Part model, mm, in its own coordinate system. A direction names the side the tool comes from. Round coordinates to 2 decimals unless told otherwise and drop trailing zeros. Write each loop counter-clockwise with the first axis right and the second up, starting at its lowest first coordinate (ties: lowest second). Pieces come first, ordered by that corner, then holes. Notation, with made-up numbers: M -2.5,86.25 L 29.5,86.25 A26 ccw 29.5,102.25 Z; hole C 34.25,8.25 d4. An arc over 180 degrees is marked long. Answer as a JSON object with one key per item and string values. Group by question number.
1. Band-saw the part on A-A, the plane y = 40.5. Write the cut outline in (x, z), plus the area to 3 significant figures.
2. Drill centre lines: line 1 (Y direction, x = -40, z = 34); line 2 (Y direction, x = 34.5, z = 29.5). Where is each one in solid material? Low to high. Write a range as from..to.
3. Two-plate mould, pull along X, no slides. Class faces 1 (the face through (40, -40, 32)), 2 (the face through (44, -1, 21)), 3 (the face through (-1, -44, 21)): +X half, -X half, draft (parallel to the pull), parting line (faces both ways), or undercut.
4. Band-saw the part on D-D, the plane z = 38.5. Write the cut outline in (x, y).
5. Band-saw the part on B-B, the plane x = 22.5. Write the cut outline in (y, z), plus the area to 3 significant figures.
6. Band-saw the part on C-C, the plane z = 9.5. Write the cut outline in (x, y), plus the area to 3 significant figures.
7. Which spindle directions (+Z, -Z, +X, -X, +Y, -Y) get a long thin tool onto all of the face, cutting with end or side? Do faces 4 (the face through (37.19, -40, 22)), 5 (the face through (-1, 44, 21)). Say none if no direction does.
8. Drop a flat-ended pin along its axis: pin 1 (0.8 mm diameter, centred on x = -40.5, y = -40.5, fed in from +Z). Give the stop position or say it passes through.
from build123d import *

# Parameters (mm, degrees)
SKETCH_W        = 88
SKETCH_H        = 88
PAD_DEPTH       = 42
SKETCH001_W     = 84
SKETCH001_H     = 84
POCKET_DEPTH    = 39
SKETCH002_W     = 5
SKETCH002_H     = 5
PAD001_DEPTH    = 39
SKETCH003_R     = 1.25
POCKET001_DEPTH = 10


with BuildPart() as part:
    # Sketch → Pad (new body)
    with BuildSketch(Plane.XY):
        Rectangle(SKETCH_W, SKETCH_H)
    extrude(amount=PAD_DEPTH)

    # Sketch001 (on Face6 of Pad) → Pocket (cut)
    with BuildSketch(Plane.XY.offset(42)):
        Rectangle(SKETCH001_W, SKETCH001_H)
    extrude(amount=-POCKET_DEPTH, mode=Mode.SUBTRACT)

    # Sketch002 (on Face11 of Pocket) → Pad001 (join)
    with BuildSketch(Plane.XY.offset(3)):
        with Locations((-39.556091, 39.69)):
            Rectangle(SKETCH002_W, SKETCH002_H)
        with Locations((-39.69, -39.556091)):
            Rectangle(SKETCH002_W, SKETCH002_H)
    pad001 = extrude(amount=PAD001_DEPTH)

    # Mirrored: Pad001 across Sketch002 V_Axis
    add(pad001.mirror(Plane(origin=(0, 0, 3), x_dir=(0, 0, 1), z_dir=(1, 0, 0))))

    # Sketch003 (on Face6 of Mirrored) → Pocket001 (cut)
    with BuildSketch(Plane.XY.offset(42)):
        with Locations((-40, 40.5)):
            Circle(SKETCH003_R)
        with Locations((-40, -40.5)):
            Circle(SKETCH003_R)
    pocket001 = extrude(amount=-POCKET001_DEPTH, mode=Mode.SUBTRACT)

    # Mirrored001: Pocket001 across Sketch003 V_Axis
    add(pocket001.mirror(Plane(origin=(0, 0, 42), x_dir=(0, 0, 1), z_dir=(1, 0, 0))), mode=Mode.SUBTRACT)


solid = part.part
Worked answers:
{
 "1": {"outline": "M -44,0 L 44,0 L 44,42 L 41.25,42 L 41.25,32 L 38.75,32 L 38.75,42 L 37.06,42 L 37.06,3 L -37.06,3 L -37.06,42 L -38.75,42 L -38.75,32 L -41.25,32 L -41.25,42 L -44,42 Z", "area": "756 mm^2"},
 "2": {"line 1": "y = -44..-41.75, -39.25..-37.06, 37.19..39.25, 41.75..44", "line 2": "y = -44..-42, 42..44"},
 "3": {"face 1": "undercut", "face 2": "+X half", "face 3": "draft"},
 "4": {"outline": "M -44,-44 L 44,-44 L 44,44 L -44,44 Z; hole M -42,-37.06 L -37.19,-37.06 L -37.19,-42 L 37.19,-42 L 37.19,-37.06 L 42,-37.06 L 42,37.19 L 37.06,37.19 L 37.06,42 L -37.06,42 L -37.06,37.19 L -42,37.19 Z; hole C -40,-40.5 d2.5; hole C -40,40.5 d2.5; hole C 40,-40.5 d2.5; hole C 40,40.5 d2.5"},
 "5": {"outline": "M -44,0 L 44,0 L 44,42 L 42,42 L 42,3 L -42,3 L -42,42 L -44,42 Z", "area": "420 mm^2"},
 "6": {"outline": "M -44,-44 L 44,-44 L 44,44 L -44,44 Z; hole M -42,-37.06 L -37.19,-37.06 L -37.19,-42 L 37.19,-42 L 37.19,-37.06 L 42,-37.06 L 42,37.19 L 37.06,37.19 L 37.06,42 L -37.06,42 L -37.06,37.19 L -42,37.19 Z", "area": "783 mm^2"},
 "7": {"face 4": "+Z", "face 5": "+Z, -Z, +X, -X, +Y"},
 "8": {"pin 1": "stops at z = 32"}
}
